Here's the drawing with two shaded views (mm, measured from the low corner). I have some questions. Give positions to 0.01 mm unless a question says otherwise; leave off trailing zeros. Loops run counter-clockwise (first coordinate to the right, second up) from the corner with the lowest first, then second, coordinate; pieces in that order, holes last. Notation, with made-up numbers: (60.25, 88) - (108.25, 88) arc R30 ccw to (108.25, 110) - close; hole circle Ø10 at (67.25, -5.5). An arc over 180 degrees is marked (long way). Use a Markdown table: item, result. Add a question column.
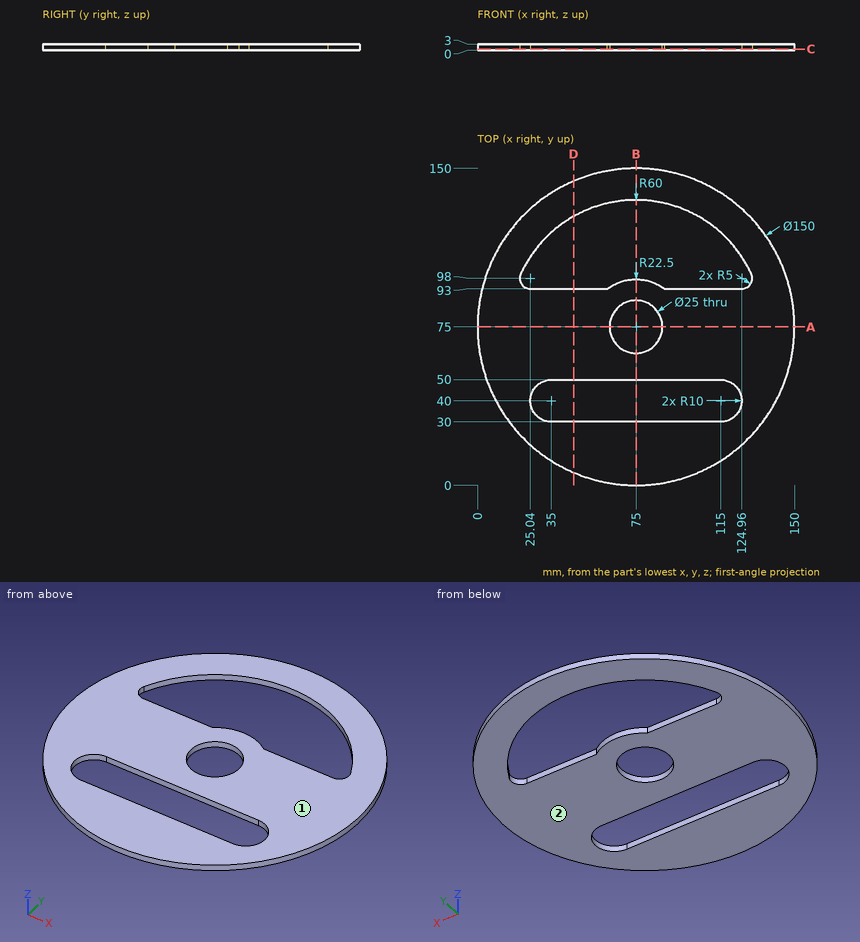
1. Suppose I cut it at B-B (x = 75). List the corners of the cut face in (y, z) for me, and give its area (4 significant figures).
2. Suppose I cut it at A-A (y = 75). List the corners of the cut face in (x, z) for me.
3. Please list where these lines run through material, in increasing order: line 1 along Y through (x, z) = (75, 1.45); line 2 along X through (y, z) = (74.5, 1.95); line 3 along Y through (x, z) = (36.5, 1). Write a range as [from, to].
4. Will these pins go through, and if not, where does the flat tip stop? P1, Ø1.5, axis at x = 78, y = 50, coming from the -Z side; P2, Ø0.9, axis at x = 66, z = 2, coming from the -Y side; P3, Ø0.9, axis at x = 48, z = 2, coming from the +Y side; P4, Ø1, axis at y = 99, z = 0.5, coming from the -X side.
5. Suppose I cut it at C-C (z = 0.55). List the corners of the cut face in (x, y) for me.
6. Suppose I cut it at D-D (x = 45.5). List the corners of the cut face in (y, z) for me.
7. If we mould it in two halves opening along Z, with no side actions, what happens to the marked faces 1 and 2? For each: released by +Z, released by -Z, zero draft, split by the parting line, or undercut.
Results below:
| question | item | result |
|---|---|---|
| 1 | outline | (0, 0) - (30, 0) - (30, 3) - (0, 3) - close; (50, 0) - (62.5, 0) - (62.5, 3) - (50, 3) - close; (87.5, 0) - (97.5, 0) - (97.5, 3) - (87.5, 3) - close; (135, 0) - (150, 0) - (150, 3) - (135, 3) - close |
| 1 | area | 202.5 mm² |
| 2 | outline | (0, 0) - (62.5, 0) - (62.5, 3) - (0, 3) - close; (87.5, 0) - (150, 0) - (150, 3) - (87.5, 3) - close |
| 3 | line 1 | [0, 30], [50, 62.5], [87.5, 97.5], [135, 150] |
| 3 | line 2 | [0, 62.51], [87.49, 150] |
| 3 | line 3 | [10.64, 30], [50, 93], [121.02, 139.36] |
| 4 | P1 | z = 0 |
| 4 | P2 | y = 0.49 |
| 4 | P3 | y = 145.14 |
| 4 | P4 | x = 3.78 |
| 5 | outline | circle Ø150 at (75, 75); hole (20.5, 100.09) arc R5 ccw to (25.04, 93) - (61.5, 93) arc R22.5 cw to (88.5, 93) - (124.96, 93) arc R5 ccw to (129.5, 100.09) arc R60 ccw to start; hole (35, 30) - (115, 30) arc R10 ccw to (115, 50) - (35, 50) arc R10 ccw to start; hole circle Ø25 at (75, 75) |
| 6 | outline | (6.05, 0) - (30, 0) - (30, 3) - (6.05, 3) - close; (50, 0) - (93, 0) - (93, 3) - (50, 3) - close; (127.25, 0) - (143.95, 0) - (143.95, 3) - (127.25, 3) - close |
| 7 | face 1 | released by +Z |
| 7 | face 2 | released by -Z |
